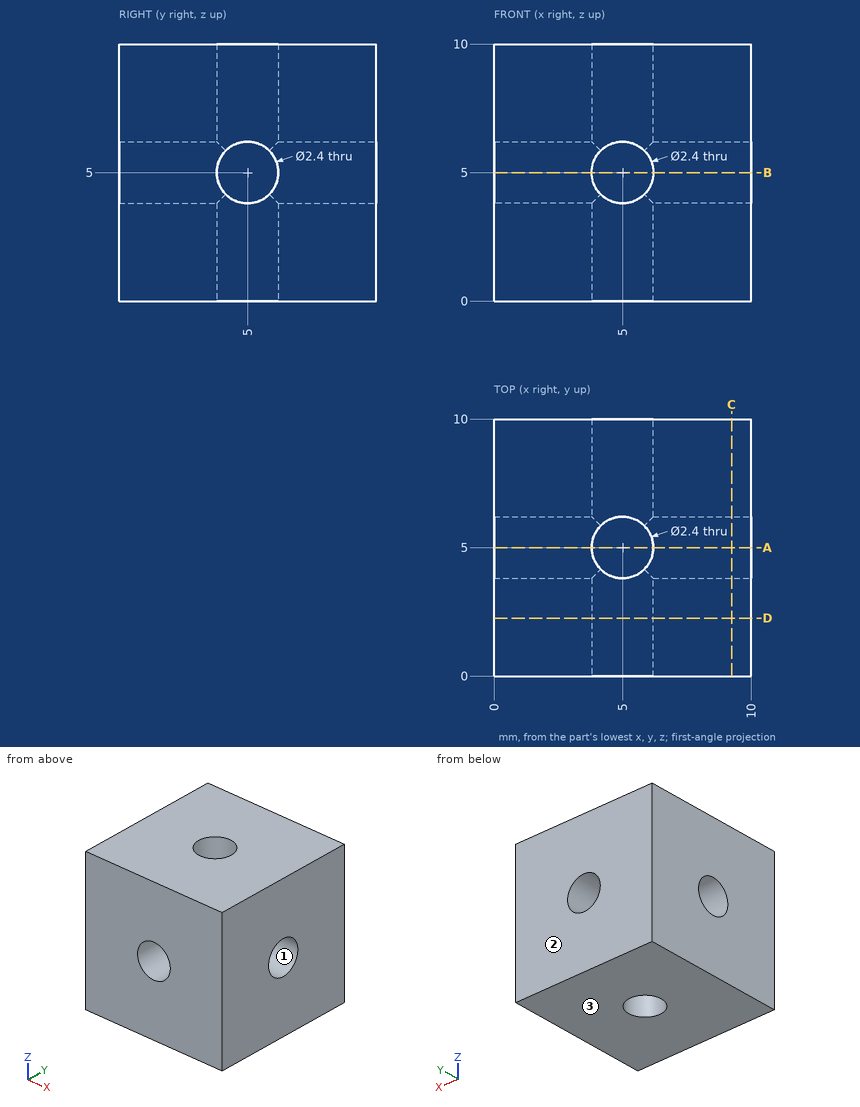
Design review of the part shown in the three views and the two pictorial views. Dimensions are in mm from the part's minimum x, y and z. Round coordinates to 2 decimals unless told otherwise and drop trailing zeros. Order: outer loops, then holes, each group sorted by start corner. A loop starts at its lowest first (then second) coordinate and runs counter-clockwise, first axis right, second up.
(1) Wall thickness on L1, parallel to Z at x = 3.3, y = 5: over which ranges is the line inside the solid? List them lowest first.
Working result:
L1: z = 0 to 3.8, 6.2 to 10
(2) Take a section at A-A, the plane y = 5. State the section outline as (x, z) points.
Working result:
outline: (0, 0) - (3.8, 0) - (3.8, 3.8) - (0, 3.8) - close; (0, 6.2) - (3.8, 6.2) - (3.8, 10) - (0, 10) - close; (6.2, 0) - (10, 0) - (10, 3.8) - (6.2, 3.8) - close; (6.2, 6.2) - (10, 6.2) - (10, 10) - (6.2, 10) - close
(3) For P1, Ø1.4, axis at y = 5, z = 5, coming from the +X side; P2, Ø3, axis at x = 8, z = 1.5, coming from the -Y side, all flat-tipped, find the tip position at first contact; note any pin that passes through.
Working result:
P1: passes through
P2: stops at y = 0
(4) Mouldability with a two-part tool opening along Y and no side actions: class the marked faces 1, 2 and 3 as released by +Y, released by -Y, zero draft, split by the parting line, or undercut.
Working result:
face 1: undercut
face 2: released by +Y
face 3: zero draft
(5) Take a section at C-C, the plane x = 9.25. State the section outline as (y, z) points, plus the area to 3 significant figures.
Working result:
outline: (0, 0) - (10, 0) - (10, 10) - (0, 10) - close; hole circle Ø2.4 at (5, 5)
area: 95.5 mm2
